Could you check a few things on this drawing? It's one solid part, dimensions in mm from its lowest x, y, z. A direction names the side the tool comes from. Coordinates: 2 decimals unless noted, no trailing zeros. Write each loop counter-clockwise with the first axis right and the second up, starting at its lowest first coordinate (ties: lowest second). Pieces come first, ordered by that corner, then holes. Notation, with made-up numbers: (45.5, 81) - (80.5, 81) arc R23 ccw to (80.5, 108) - close; hole circle Ø8 at (-20, 61.5). An arc over 180 degrees is marked (long way). Write item = value, one per line. Start each with the question number.
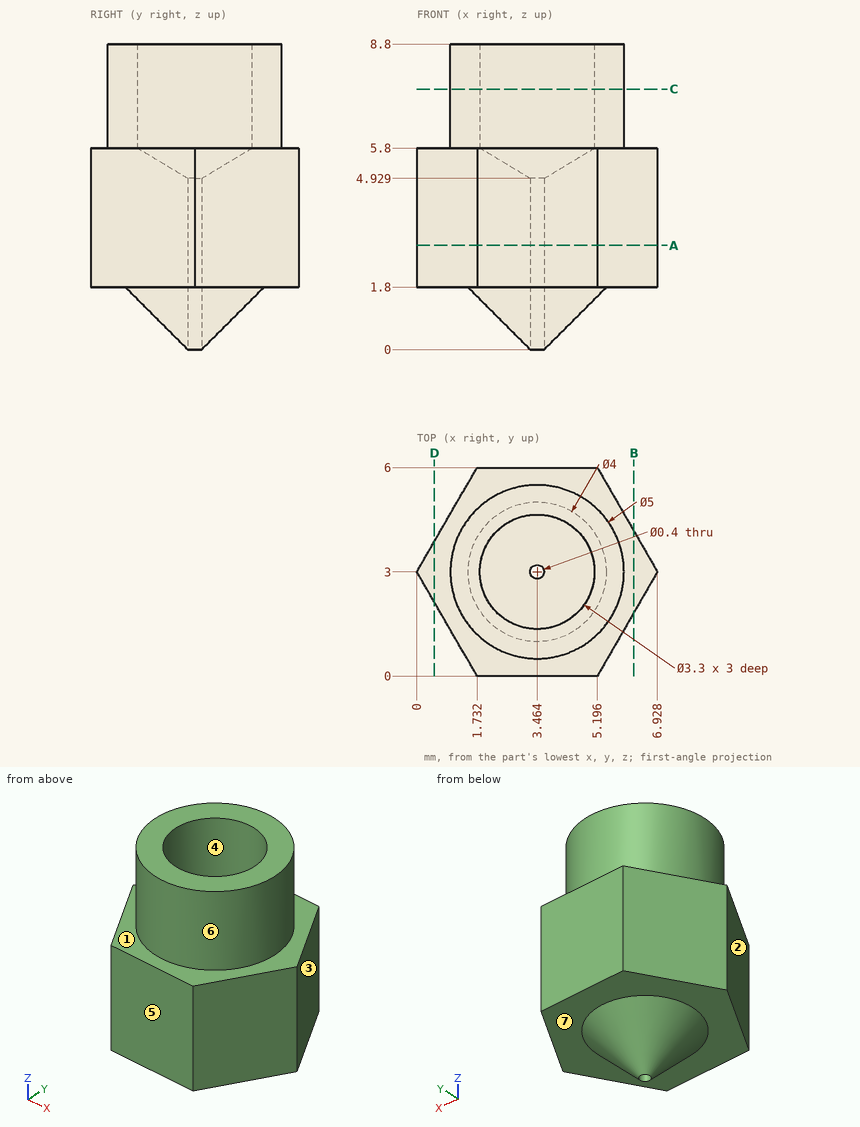
1) For P1, Ø2, axis at y = 1.5, z = 7, coming from the +X side, with a flat end and sliding along its axis, tell me the tip position at first contact or that it passes through.
2) Suppose I cut it at C-C on z = 7.5. Please give me the cut outline in (x, y).
3) Which directions (+Z, -Z, +X, -X, +Y, -Y) give clear straight access to the entire face, cutting with the end or side of a thin tool? Please do the marked faces 5, 6 and 7.
4) If I drill on probe 1 along Z at (x, y) = (3.5, 5.75); probe 2 along Y at (x, z) = (2, 7.5) (1 decimal); probe 3 along X at (y, z) = (3.5, 5.5), over which ranges is the centre line in solid material (lowest first)? Write a range as [from, to].
5) Suppose I cut it at A-A on z = 3. Please give me the cut outline in (x, y).
6) Suppose I cut it at B-B on x = 6.25. Please give me the cut outline in (y, z) (1 decimal).
7) Thinking about a two-plate mould opening in X: for the marked faces 1, 2, 3 and 4, which applies, +X half, -X half, draft (parallel to the pull), parting line (faces both ways), or undercut?
8) Suppose I cut it at D-D on x = 0.5. Please give me the cut outline in (y, z).
Reply:
q1.P1 = 5.91
q2.outline = circle Ø5 at (3.46, 3); hole circle Ø3.3 at (3.46, 3)
q3.face_5 = +Z, -Z, +X, -X, -Y
q3.face_6 = +Z
q3.face_7 = -Z
q4.probe_1 = [1.8, 5.8]
q4.probe_2 = [1, 2.2], [3.8, 5]
q4.probe_3 = [0.29, 2.43], [4.5, 6.64]
q5.outline = (0, 3) - (1.73, 0) - (5.2, 0) - (6.93, 3) - (5.2, 6) - (1.73, 6) - close; hole circle Ø0.4 at (3.46, 3)
q6.outline = (1.8, 1.8) - (4.2, 1.8) - (4.2, 5.8) - (1.8, 5.8) - close
q7.face_1 = draft
q7.face_2 = -X half
q7.face_3 = +X half
q7.face_4 = undercut
q8.outline = (2.13, 1.8) - (3.87, 1.8) - (3.87, 5.8) - (2.13, 5.8) - close
